For this review, use the dimensioned drawing (mm, ordinates from the lowest corner) and the shaded views. Give positions to 0.01 mm unless a question says otherwise; leave off trailing zeros. Loops run counter-clockwise (first coordinate to the right, second up) from the corner with the lowest first, then second, coordinate; pieces in that order, holes last. Notation, with made-up numbers: (5.25, 52.25) - (37.25, 52.25) arc R19 ccw to (37.25, 89.25) - close; hole circle Ø9 at (-9, 16.25). An arc over 180 degrees is marked (long way). Put each result on its own line as item: value.
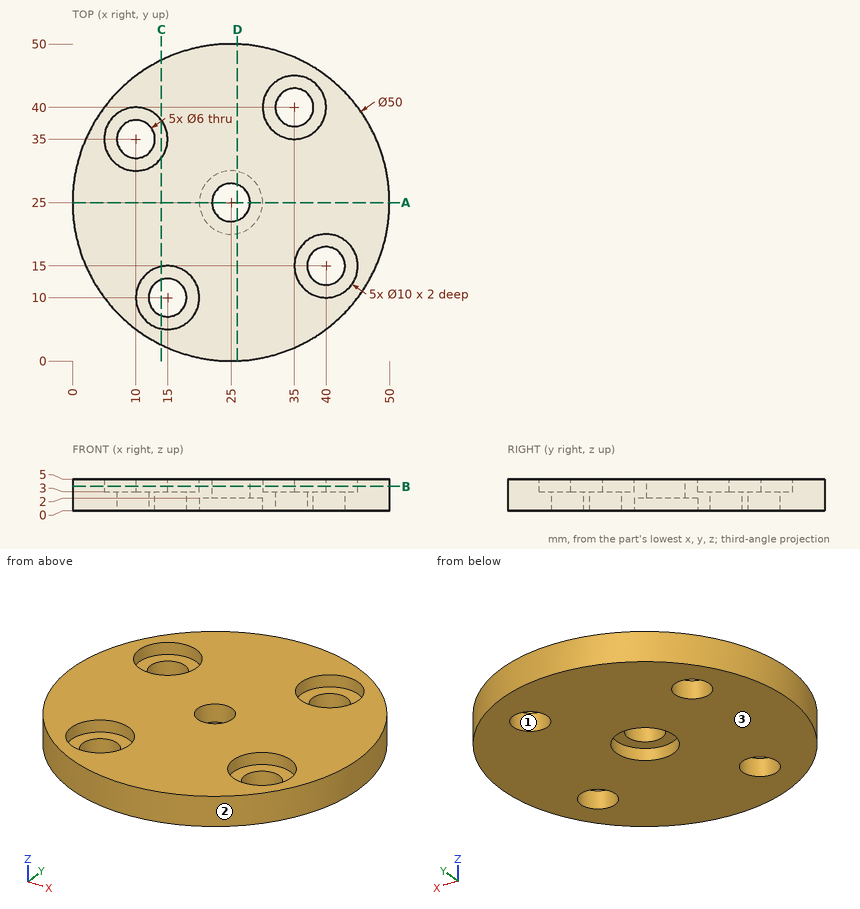
1) Take a section at A-A on y = 25. State the section outline as (x, z) points, and give its area (3 significant figures).
Geometry check:
outline: (0, 0) - (20, 0) - (20, 2) - (22, 2) - (22, 5) - (0, 5) - close; (28, 2) - (30, 2) - (30, 0) - (50, 0) - (50, 5) - (28, 5) - close
area: 212 mm²
2) Insertion check: pin 1 Ø1 at (y, z) = (40, 2) entering from -X; pin 2 Ø3 at (x, y) = (12, 32.5) entering from +Z; pin 3 Ø5 at (x, y) = (23.5, 26.5) entering from -Z. Each pin has a flat end and moves straight along its axis. Give the tip position at first contact, or say it passes through.
Geometry check:
pin 1: stops at x = 4.63
pin 2: stops at z = 3
pin 3: stops at z = 2
3) Take a section at B-B on z = 3.85. State the section outline as (x, y) points, and give its area (3 significant figures).
Geometry check:
outline: circle Ø50 at (25, 25); hole circle Ø10 at (10, 35); hole circle Ø10 at (15, 10); hole circle Ø6 at (25, 25); hole circle Ø10 at (35, 40); hole circle Ø10 at (40, 15)
area: 1,620 mm²
4) Take a section at D-D on x = 26. State the section outline as (y, z) points.
Geometry check:
outline: (0.02, 0) - (20.1, 0) - (20.1, 2) - (22.17, 2) - (22.17, 5) - (0.02, 5) - close; (27.83, 2) - (29.9, 2) - (29.9, 0) - (49.98, 0) - (49.98, 5) - (27.83, 5) - close
5) Draft analysis for pull direction X (two halves, no side actions). For the marked faces 1, 2 and 3, state which applies: pulls with the +X half, pulls with the -X half, needs draft (parallel to the pull), parting line crosses it, or undercut.
Geometry check:
face 1: undercut
face 2: parting line crosses it
face 3: needs draft
6) Wall thickness on line 1 (Y direction, x = 40, z = 2.7); line 2 (Y direction, x = 45, z = 1.3); line 3 (Y direction, x = 19.5, z = 3.45): over which ranges is each line inside the solid? List them lowest first.
Geometry check:
line 1: y = 5 to 12, 18 to 45
line 2: y = 10 to 40
line 3: y = 0.61 to 7.82, 12.18 to 49.39
7) Take a section at C-C on x = 14. State the section outline as (y, z) points.
Geometry check:
outline: (2.55, 0) - (7.17, 0) - (7.17, 3) - (5.1, 3) - (5.1, 5) - (2.55, 5) - close; (12.83, 0) - (47.45, 0) - (47.45, 5) - (38, 5) - (38, 3) - (32, 3) - (32, 5) - (14.9, 5) - (14.9, 3) - (12.83, 3) - close
